Could you check a few things on this drawing? It's one solid part, dimensions in mm from its lowest x, y, z. Give positions to 0.01 mm unless a question says otherwise; leave off trailing zeros. Loops run counter-clockwise (first coordinate to the right, second up) from the corner with the lowest first, then second, coordinate; pieces in that order, holes last. Notation, with made-up numbers: (42, -37.5) - (68, -37.5) arc R10 cw to (68, -26.5) - close; hole circle Ø4 at (77.5, 74.5). An arc over 180 degrees is marked (long way). Use CSV: the item, a comma, the result in double quotes.
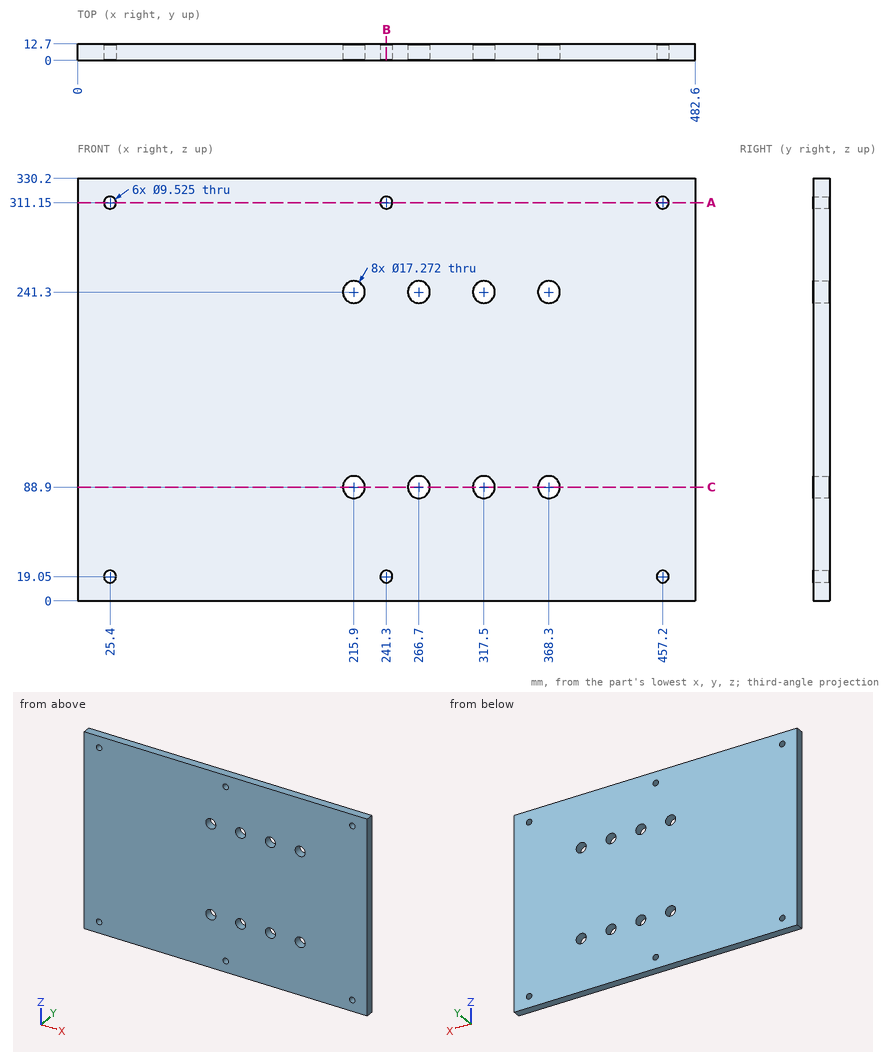
1) Suppose I cut it at C-C (z = 88.9). Please give me the cut outline in (x, y).
Answer below:
outline,"(0, 0) - (207.26, 0) - (207.26, 12.7) - (0, 12.7) - close; (224.54, 0) - (258.06, 0) - (258.06, 12.7) - (224.54, 12.7) - close; (275.34, 0) - (308.86, 0) - (308.86, 12.7) - (275.34, 12.7) - close; (326.14, 0) - (359.66, 0) - (359.66, 12.7) - (326.14, 12.7) - close; (376.94, 0) - (482.6, 0) - (482.6, 12.7) - (376.94, 12.7) - close"
2) Suppose I cut it at A-A (z = 311.15). Please give me the cut outline in (x, y).
Answer below:
outline,"(0, 0) - (20.64, 0) - (20.64, 12.7) - (0, 12.7) - close; (30.16, 0) - (236.54, 0) - (236.54, 12.7) - (30.16, 12.7) - close; (246.06, 0) - (452.44, 0) - (452.44, 12.7) - (246.06, 12.7) - close; (461.96, 0) - (482.6, 0) - (482.6, 12.7) - (461.96, 12.7) - close"
3) Suppose I cut it at B-B (x = 241.3). Please give me the cut outline in (y, z), plus the area to 3 significant figures.
Answer below:
outline,"(0, 0) - (12.7, 0) - (12.7, 14.29) - (0, 14.29) - close; (0, 23.81) - (12.7, 23.81) - (12.7, 306.39) - (0, 306.39) - close; (0, 315.91) - (12.7, 315.91) - (12.7, 330.2) - (0, 330.2) - close"
area,"3,950 mm2"
4) I need wall thicknesses on line 1 along X through (y, z) = (3, 311.15); line 2 along X through (y, z) = (9, 241.3); line 3 along Z through (x, y) = (241.3, 5.75). Which ranges of each line are inside material? Lowest first, please.
Answer below:
line 1,"x = 0 to 20.64, 30.16 to 236.54, 246.06 to 452.44, 461.96 to 482.6"
line 2,"x = 0 to 207.26, 224.54 to 258.06, 275.34 to 308.86, 326.14 to 359.66, 376.94 to 482.6"
line 3,"z = 0 to 14.29, 23.81 to 306.39, 315.91 to 330.2"
5) I'm going to push a flat-ended pin straight in: P1, Ø15.5, axis at x = 368.3, z = 88.9, coming from the +Y side. Where does the tip first touch, or does it pass through?
Answer below:
P1,"passes through"
